from build123d import *

# Parameters (mm, degrees)
F1_DEPTH = 25
F2_W     = 40
F2_H     = 40
F3_DEPTH = 7.5
F4_R     = 10
F5_DEPTH = 15
F6_R     = 20


with BuildPart() as f1:
    # F0 (on Front) → F1 (new body, symmetric)
    with BuildSketch(Plane.XZ):
        Polygon((27.5, 7.5), (-27.5, 7.5), (-27.5, -7.5), (-17.5, -7.5), (-17.5, -2.5), (17.5, -2.5), (17.5, -7.5), (27.5, -7.5), align=None)
    extrude(amount=F1_DEPTH, both=True)

    # F2 (on Right) → F3 (join, symmetric)
    with BuildSketch(Plane.YZ):
        with Locations((5, 27.5)):
            Rectangle(F2_W, F2_H)
    extrude(amount=F3_DEPTH, both=True)

    # F4 (on face) → F5 (cut, through all)
    with BuildSketch(Plane.YZ.offset(7.5)):
        with Locations((5, 27.5)):
            Circle(F4_R)
    extrude(amount=-F5_DEPTH, mode=Mode.SUBTRACT)

    # F6
    f6_edges = [f1.edges().sort_by_distance(p)[0] for p in [
        (0, 25, 47.5),
    ]]
    fillet(f6_edges, radius=F6_R)


solid = f1.part
The model under review builds one solid part; all positions refer to its coordinate system, in mm. A direction names the side the tool comes from. Round coordinates to 2 decimals unless told otherwise and drop trailing zeros. Loops run counter-clockwise (first coordinate to the right, second up) from the corner with the lowest first, then second, coordinate; pieces in that order, holes last. Notation, with made-up numbers: M -22.5,76.5 L 25.5,76.5 A14 cw 25.5,88.5 Z; hole C 31,41.5 d7. An arc over 180 degrees is marked long. Answer as CSV lines item,"result".
1. For faces 5 (the face through (0, 0, -2.5)), 6 (the face through (0, -15, 27)), 7 (the face through (7.5, -4.2, 32.2)), 8 (the face through (-7.5, -4.2, 32.2)), list the 3-axis set-ups (+Z, -Z, +X, -X, +Y, -Y) from which the entire face can be reached by the end or side of a thin tool; tool diameter is ignored.
Outcome:
face 5,"-Z, +Y, -Y"
face 6,"+Z, +X, -X, -Y"
face 7,"+Z, +X, +Y, -Y"
face 8,"+Z, -X, +Y, -Y"
2. Insertion check: pin 1 Ø10.5 at (x, y) = (8.5, 9) entering from -Z; pin 2 Ø5 at (y, z) = (-6, 26.5) entering from +X; pin 3 Ø3 at (x, z) = (2.5, 31.5) entering from -Y; pin 4 Ø12 at (y, z) = (5, 27.5) entering from +X. Each pin has a flat end and moves straight along its axis. Give the tip position at first contact, or say it passes through.
Outcome:
pin 1,"stops at z = -2.5"
pin 2,"stops at x = 7.5"
pin 3,"stops at y = -15"
pin 4,"passes through"
3. We need section A-A (y = -1). Give the boundary of the cut face in (x, z), plus the area to 3 significant figures.
Outcome:
outline,"M -27.5,-7.5 L -17.5,-7.5 L -17.5,-2.5 L 17.5,-2.5 L 17.5,-7.5 L 27.5,-7.5 L 27.5,7.5 L 7.5,7.5 L 7.5,19.5 L -7.5,19.5 L -7.5,7.5 L -27.5,7.5 Z; M -7.5,35.5 L 7.5,35.5 L 7.5,47.5 L -7.5,47.5 Z"
area,"1,010 mm2"
4. We need section C-C (x = 23). Give the boundary of the cut face in (y, z).
Outcome:
outline,"M -25,-7.5 L 25,-7.5 L 25,7.5 L -25,7.5 Z"
5. We need section D-D (y = 20). Give the boundary of the cut face in (x, z).
Outcome:
outline,"M -27.5,-7.5 L -17.5,-7.5 L -17.5,-2.5 L 17.5,-2.5 L 17.5,-7.5 L 27.5,-7.5 L 27.5,7.5 L 7.5,7.5 L 7.5,40.73 L -7.5,40.73 L -7.5,7.5 L -27.5,7.5 Z"
6. We need section B-B (y = -6.5). Give the boundary of the cut face in (x, z), plus the area to 3 significant figures.
Outcome:
outline,"M -27.5,-7.5 L -17.5,-7.5 L -17.5,-2.5 L 17.5,-2.5 L 17.5,-7.5 L 27.5,-7.5 L 27.5,7.5 L 7.5,7.5 L 7.5,47.5 L -7.5,47.5 L -7.5,7.5 L -27.5,7.5 Z"
area,"1,250 mm2"
7. To check wall thickness, follow L1, parallel to Y at x = 0, z = 27; L2, parallel to X at y = 20, z = -3; L3, parallel to Z at x = -8, y = -3. State the ranges of each line that lie inside material, in increasing order. Write a range as [from, to].
Outcome:
L1,"y = [-15, -4.99], [14.99, 25]"
L2,"x = [-27.5, -17.5], [17.5, 27.5]"
L3,"z = [-2.5, 7.5]"
8. Draft analysis for pull direction Z (two halves, no side actions). For faces 1 (the face through (0, -25, 2)), 2 (the face through (-23, 0, -7.5)), 3 (the face through (0, -5, 47.5)), 4 (the face through (0.105, 9.614, 18.628)), state which applies: pulls with the +Z half, pulls with the -Z half, needs draft (parallel to the pull), parting line crosses it, or undercut.
Outcome:
face 1,"needs draft"
face 2,"pulls with the -Z half"
face 3,"pulls with the +Z half"
face 4,"undercut"
